Design review of the part built by this model. Coordinates are the model's own, in mm. Face numbers are marked on the shaded views. Coordinates: 2 decimals unless noted, no trailing zeros. Loops run counter-clockwise (first coordinate to the right, second up) from the corner with the lowest first, then second, coordinate; pieces in that order, holes last. Notation, with made-up numbers: (20.25, 14) -> (53.25, 14) arc R25 cw to (53.25, 49) -> close; hole circle Ø9 at (78.5, 34.5). An arc over 180 degrees is marked (long way). Use a Markdown table: item, result. Add a question column.
Q1. Take a section at D-D on y = 28. Write out the cut boundary in (x, z).
Q2. Take a section at B-B on y = -28. Write out the cut boundary in (x, z), plus the area to 3 significant figures.
Q3. For probe 1 along Y at (x, z) = (27, -3.1); probe 2 along Y at (x, z) = (-27, -0.9); probe 3 along Z at (x, y) = (0, -18), list the stretches that pass through material, from the lowest coordinate up.
Q4. Take a section at C-C on x = 16.5. Write out the cut boundary in (y, z).
Q5. Take a section at A-A on x = 27. Write out the cut boundary in (y, z).
Q6. Clearance check with flat-ended pins moving along their axes: pin 1 Ø4 at (x, y) = (-28.06, -28) entering from -Z; pin 2 Ø4 at (x, y) = (23.5, -21.5) entering from -Z; pin 3 Ø8 at (x, y) = (5, -10) entering from +Z; pin 4 Ø1 at (x, z) = (-2, -24) entering from +Y. State where each tip first meets the part, or that it passes through.
Q7. Draft analysis for pull direction Z (two halves, no side actions). For the marked faces 1, 2 and 3, state which applies: pulls with the +Z half, pulls with the -Z half, needs draft (parallel to the pull), parting line crosses it, or undercut.
from build123d import *

# Parameters (mm, degrees)
SKETCH1_R           = 21
BOSS_EXTRUDE1_DEPTH = 8
SKETCH2_R           = 2
CUT_EXTRUDE1_DEPTH  = 10
SKETCH4_R           = 1.1
CUT_EXTRUDE2_DEPTH  = 10
SKETCH5_R           = 1.1
CUT_EXTRUDE3_DEPTH  = 10
SKETCH11_W          = 64
SKETCH11_H          = 66
BOSS_EXTRUDE3_DEPTH = 4
FILLET12_R          = 1
SKETCH16_W          = 14
SKETCH16_H          = 5
CUT_EXTRUDE7_DEPTH  = 22
SKETCH17_R          = 21
CUT_EXTRUDE9_DEPTH  = 8
SKETCH18_R          = 2.1
CUT_EXTRUDE10_DEPTH = 12
SKETCH19_R          = 4
BOSS_EXTRUDE4_DEPTH = 20


with BuildPart() as part:
    # Sketch1 → Boss-Extrude1 (new body)
    with BuildSketch(Plane.XY):
        Circle(SKETCH1_R)
    extrude(amount=BOSS_EXTRUDE1_DEPTH)

    # Sketch2 → Cut-Extrude1 (cut)
    with BuildSketch(Plane(origin=(0, 0, 0), x_dir=(-1, 0, 0), z_dir=(0, 0, -1))):
        Circle(SKETCH2_R)
    extrude(amount=-CUT_EXTRUDE1_DEPTH, mode=Mode.SUBTRACT)

    # Sketch4 → Cut-Extrude2 (cut)
    with BuildSketch(Plane(origin=(0, 0, 0), x_dir=(-1, 0, 0), z_dir=(0, 0, -1))):
        with Locations((16, 0)):
            Circle(SKETCH4_R)
    extrude(amount=-CUT_EXTRUDE2_DEPTH, mode=Mode.SUBTRACT)

    # Sketch5 → Cut-Extrude3 (cut)
    with BuildSketch(Plane(origin=(0, 0, 0), x_dir=(-1, 0, 0), z_dir=(0, 0, -1))):
        with Locations((-16, 0)):
            Circle(SKETCH5_R)
    extrude(amount=-CUT_EXTRUDE3_DEPTH, mode=Mode.SUBTRACT)

    # Sketch11 → Boss-Extrude3 (add)
    with BuildSketch(Plane(origin=(0, 0, 0), x_dir=(-1, 0, 0), z_dir=(0, 0, -1))):
        Rectangle(SKETCH11_W, SKETCH11_H)
    extrude(amount=BOSS_EXTRUDE3_DEPTH)

    # Fillet12
    fillet12_edges = [part.edges().sort_by_distance(p)[0] for p in [
        (-32, 0, -4),
        (0, 33, -4),
        (32, 0, -4),
        (0, -33, -4),
    ]]
    fillet(fillet12_edges, radius=FILLET12_R)

    # Sketch16 → Cut-Extrude7 (cut)
    with BuildSketch(Plane(origin=(0, 0, -4), x_dir=(-1, 0, 0), z_dir=(0, 0, -1))):
        with Locations((-13.170947401, 26.5)):
            Rectangle(SKETCH16_W, SKETCH16_H)
    extrude(amount=-CUT_EXTRUDE7_DEPTH, mode=Mode.SUBTRACT)

    # Sketch17 → Cut-Extrude9 (cut)
    with BuildSketch(Plane.XY.offset(8)):
        Circle(SKETCH17_R)
    extrude(amount=-CUT_EXTRUDE9_DEPTH, mode=Mode.SUBTRACT)

    # Sketch18 → Cut-Extrude10 (cut)
    with BuildSketch(Plane(origin=(0, 0, -4), x_dir=(-1, 0, 0), z_dir=(0, 0, -1))):
        with Locations((-27, 28)):
            Circle(SKETCH18_R)
        with Locations((-27, -28)):
            Circle(SKETCH18_R)
        with Locations((28.056628896, -28)):
            Circle(SKETCH18_R)
        with Locations((27, 28)):
            Circle(SKETCH18_R)
    extrude(amount=-CUT_EXTRUDE10_DEPTH, mode=Mode.SUBTRACT)

    # Sketch19 → Boss-Extrude4 (add)
    with BuildSketch(Plane(origin=(0, 0, -4), x_dir=(-1, 0, 0), z_dir=(0, 0, -1))):
        Circle(SKETCH19_R)
    extrude(amount=BOSS_EXTRUDE4_DEPTH)

    # Sketch20 → Revolve1 (revolve)
    with BuildSketch(Plane(origin=(0, 0, 0), x_dir=(1, 0, 0), z_dir=(0, 1, 0))):
        with BuildLine():
            Line((0, 24), (-4, 24))
            ThreePointArc((-4, 24), (-2.828427125, 26.828427125), (0, 28))
            Line((0, 28), (0, 24))
        make_face()
    revolve(axis=Axis((0, 0, -24), (0, 0, -1)))


solid = part.part
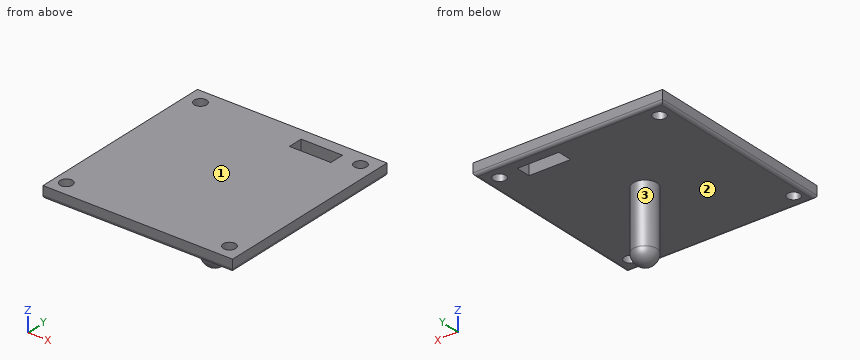
Answer list:
| question | item | result |
|---|---|---|
| 1 | outline | (-32, -3) arc R1 ccw to (-31, -4) -> (-29.1, -4) -> (-29.1, 0) -> (-32, 0) -> close; (-24.9, -4) -> (6.17, -4) -> (6.17, 0) -> (-24.9, 0) -> close; (20.17, -4) -> (24.9, -4) -> (24.9, 0) -> (20.17, 0) -> close; (29.1, -4) -> (31, -4) arc R1 ccw to (32, -3) -> (32, 0) -> (29.1, 0) -> close |
| 2 | outline | (-32, -3) arc R1 ccw to (-31, -4) -> (-30.16, -4) -> (-30.16, 0) -> (-32, 0) -> close; (-25.96, -4) -> (24.9, -4) -> (24.9, 0) -> (-25.96, 0) -> close; (29.1, -4) -> (31, -4) arc R1 ccw to (32, -3) -> (32, 0) -> (29.1, 0) -> close |
| 2 | area | 222 mm² |
| 3 | probe 1 | -32.99 to -30.1, -25.9 to 25.9, 30.1 to 32.99 |
| 3 | probe 2 | -33 to -29.81, -26.19 to 25.9, 30.1 to 33 |
| 3 | probe 3 | -4 to 0 |
| 4 | outline | (-33, -3) arc R1 ccw to (-32, -4) -> (24, -4) -> (24, 0) -> (-33, 0) -> close; (29, -4) -> (32, -4) arc R1 ccw to (33, -3) -> (33, 0) -> (29, 0) -> close |
| 5 | outline | (-33, -3) arc R1 ccw to (-32, -4) -> (-30.1, -4) -> (-30.1, 0) -> (-33, 0) -> close; (-25.9, -4) -> (25.9, -4) -> (25.9, 0) -> (-25.9, 0) -> close; (30.1, -4) -> (32, -4) arc R1 ccw to (33, -3) -> (33, 0) -> (30.1, 0) -> close |
| 6 | pin 1 | through |
| 6 | pin 2 | z = -4 |
| 6 | pin 3 | z = 0 |
| 6 | pin 4 | y = 3.71 |
| 7 | face 1 | pulls with the +Z half |
| 7 | face 2 | pulls with the -Z half |
| 7 | face 3 | needs draft |
